Geometry: final body of the model. Coordinates: model frame, mm. Give positions to 0.01 mm unless a question says otherwise; leave off trailing zeros. Write each loop counter-clockwise with the first axis right and the second up, starting at its lowest first coordinate (ties: lowest second). Pieces come first, ordered by that corner, then holes.
Q1. Pin query (flat end, axial travel): pin 1 Ø2.5 at (x, y) = (-48.53, 41.04) entering from +Z; pin 2 Ø8 at (x, y) = (-80.5, 68) entering from -Z. Return the tip coordinate at first contact, or that it passes through.
Q2. Section C-C (y = 70). Return the cut outline in (x, z), plus the area to 3 significant figures.
Q3. Section A-A (z = 0.5). Return the cut outline in (x, y) (1 decimal), plus the area to 3 significant figures.
Q4. Section B-B (x = -60). Return the cut outline in (y, z), plus the area to 3 significant figures.
Q5. Line query: line 1 (X direction, y = 65.5, z = 0.15); line 2 (X direction, y = 64, z = 0.65); line 3 (Y direction, x = -48.5, z = 1.1). Output: solid intervals per line, ascending.
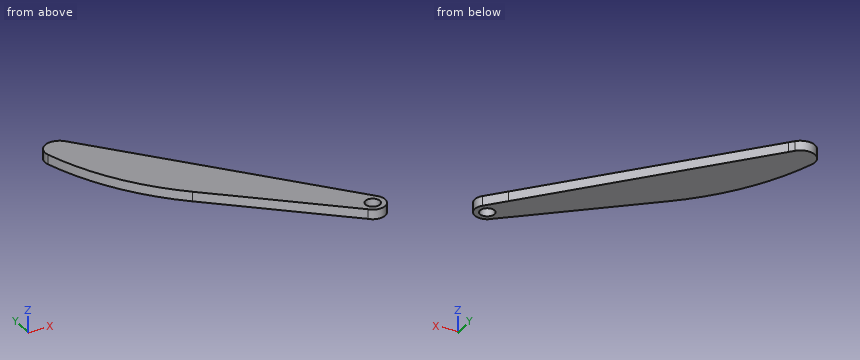
from build123d import *

# Parameters (mm, degrees)
SKETCH1_R           = 1.5
BOSS_EXTRUDE1_DEPTH = 2
FILLET1_R           = 3


with BuildPart() as part:
    # Sketch1 → Boss-Extrude1 (new body)
    with BuildSketch(Plane.XY):
        with BuildLine():
            Line((-46.636509162, 42.789020236), (-50.060973508, 46.502785938))
            Line((-50.060973508, 46.502785938), (-86.522855439, 86.04499543))
            Line((-86.522855439, 86.04499543), (-94.837872086, 95.062471017))
            ThreePointArc((-94.837872086, 95.062471017), (-88.687933444, 75.487292789), (-75.566721617, 59.712529776))
            Line((-75.566721617, 59.712529776), (-50.429932547, 39.291103519))
            ThreePointArc((-50.429932547, 39.291103519), (-46.784262496, 39.143350184), (-46.636509162, 42.789020236))
        make_face()
        with Locations((-48.533220855, 41.040061877)):
            Circle(SKETCH1_R, mode=Mode.SUBTRACT)
    extrude(amount=BOSS_EXTRUDE1_DEPTH)

    # Fillet1
    fillet1_edges = [part.edges().sort_by_distance(p)[0] for p in [
        (-94.837872086, 95.062471017, 1),
    ]]
    fillet(fillet1_edges, radius=FILLET1_R)


solid = part.part
Computed:
1. pin 1: passes through
1. pin 2: stops at z = 0
2. outline: (-85.25, 0) - (-71.73, 0) - (-71.73, 2) - (-85.25, 2) - close
2. area: 27.0 mm2
3. outline: (-92.4, 83.9) arc R53 ccw to (-75.6, 59.7) - (-50.4, 39.3) arc R2.6 ccw to (-46.6, 42.8) - (-87.3, 86.9) arc R3 ccw to start; hole circle Ø3 at (-48.5, 41)
3. area: 518 mm2
4. outline: (47.07, 0) - (57.28, 0) - (57.28, 2) - (47.07, 2) - close
4. area: 20.4 mm2
5. line 1: x = -81.64 to -67.58
5. line 2: x = -80.24 to -66.2
5. line 3: y = 38.46 to 39.54, 42.54 to 44.81
